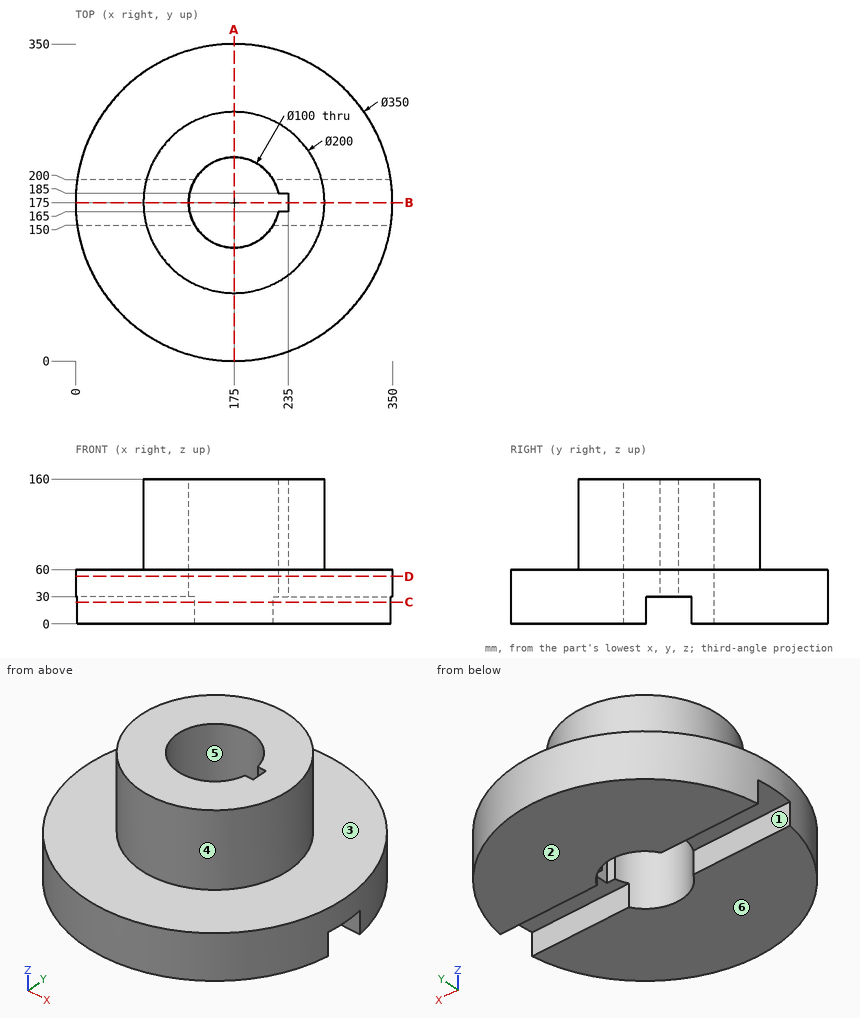
For this review, use the dimensioned drawing (mm, ordinates from the lowest corner) and the shaded views. A direction names the side the tool comes from. Round coordinates to 2 decimals unless told otherwise and drop trailing zeros. Loops run counter-clockwise (first coordinate to the right, second up) from the corner with the lowest first, then second, coordinate; pieces in that order, holes last. Notation, with made-up numbers: (35.25, -16) -> (83.25, -16) arc R20 cw to (83.25, 19) -> close; hole circle Ø10 at (-18.5, 84.25). An arc over 180 degrees is marked (long way). Write item = value, one per line. Start each with the question number.
Item 1: To check wall thickness, follow L1, parallel to X at y = 175, z = 37; L2, parallel to Y at x = 175, z = 47; L3, parallel to Y at x = 175, z = 90. State the ranges of each line that lie inside material, in increasing order.
Item 2: Take a section at C-C on z = 24. Give the boundary of the cut face in (x, y) (1 decimal).
Item 3: Take a section at A-A on x = 175. Give the boundary of the cut face in (y, z).
Item 4: Insertion check: pin 1 (5.5 mm diameter, centred on x = 231.5, z = 71.5, fed in from -Y); pin 2 (8 mm diameter, centred on x = 154.5, z = 20, fed in from -Y); pin 3 (10 mm diameter, centred on y = 227.5, z = 23, fed in from +X). Each pin has a flat end and moves straight along its axis. Give the tip position at first contact, or say it passes through.
Item 5: Mouldability with a two-part tool opening along Y and no side actions: class the marked faces 4, 5 and 6 as released by +Y, released by -Y, zero draft, split by the parting line, or undercut.
Item 6: Take a section at D-D on z = 52.5. Give the boundary of the cut face in (x, y), plus the area to 4 significant figures.
Item 7: Take a section at B-B on y = 175. Give the boundary of the cut face in (x, z).
Item 8: For the marked faces 1, 2 and 3, list the 3-axis set-ups (+Z, -Z, +X, -X, +Y, -Y) from which the entire face can be reached by the end or side of a thin tool; tool diameter is ignored.
Result:
q1.L1 = 0 to 125, 235 to 350
q1.L2 = 0 to 125, 225 to 350
q1.L3 = 75 to 125, 225 to 275
q2.outline = (1.8, 150) arc R175 ccw to (348.2, 150) -> (218.3, 150) arc R50 cw to (131.7, 150) -> close; (1.8, 200) -> (131.7, 200) arc R50 cw to (218.3, 200) -> (348.2, 200) arc R175 ccw to start
q3.outline = (0, 0) -> (125, 0) -> (125, 160) -> (75, 160) -> (75, 60) -> (0, 60) -> close; (225, 0) -> (350, 0) -> (350, 60) -> (275, 60) -> (275, 160) -> (225, 160) -> close
q4.pin_1 = 90.67
q4.pin_2 = 0.78
q4.pin_3 = 343.43
q5.face_4 = split by the parting line
q5.face_5 = undercut
q5.face_6 = zero draft
q6.outline = circle Ø350 at (175, 175); hole (223.99, 165) -> (235, 165) -> (235, 185) -> (223.99, 185) arc R50 ccw (long way) to start
q6.area = 88,150 mm²
q7.outline = (0, 30) -> (125, 30) -> (125, 160) -> (75, 160) -> (75, 60) -> (0, 60) -> close; (235, 30) -> (350, 30) -> (350, 60) -> (275, 60) -> (275, 160) -> (235, 160) -> close
q8.face_1 = -Z, +X, -X
q8.face_2 = -Z, +X, -X, +Y, -Y
q8.face_3 = +Z
